```python
from build123d import *

# Parameters (mm, degrees)
SKETCH_1_R      = 33
SKETCH_1_R_2    = 4
SKETCH_1_R_3    = 7
EXTRUDE_1_DEPTH = 10
SKETCH_1_3_R    = 33
EXTRUDE_2_DEPTH = 20


with BuildPart() as part:
    # Sketch 1 → Extrude 1 (new body)
    with BuildSketch(Plane.XY):
        with BuildLine():
            ThreePointArc((64, -136), (75.313708499, -140.686291501), (80, -152))
            Line((80, -152), (27.5, -152))
            Line((27.5, -152), (14.463080892, -104.593021426))
            ThreePointArc((14.463080892, -104.593021426), (0, -93.570368671), (-14.463080892, -104.593021426))
            Line((-14.463080892, -104.593021426), (-27.5, -152))
            Line((-27.5, -152), (-80, -152))
            ThreePointArc((-80, -152), (-75.313708499, -140.686291501), (-64, -136))
            Line((-64, -136), (-60.459937025, -136))
            ThreePointArc((-60.459937025, -136), (-51.367638325, -132.930218118), (-45.996856133, -124.977347245))
            Line((-45.996856133, -124.977347245), (-29.300488581, -64.26328342))
            ThreePointArc((-29.300488581, -64.26328342), (-29.160343249, -48.882298429), (-36.661224304, -35.453555993))
            ThreePointArc((-36.661224304, -35.453555993), (-48.195333852, -16.679622146), (-50.733420691, 5.207689026))
            ThreePointArc((-50.733420691, 5.207689026), (-51.500326923, 13.089309145), (-55.266020254, 20.05548705))
            ThreePointArc((-55.266020254, 20.05548705), (-51.548317959, 55.688646816), (-16.027753707, 51.016077878))
            ThreePointArc((-16.027753707, 51.016077878), (0, 42.978983508), (16.027753707, 51.016077878))
            ThreePointArc((16.027753707, 51.016077878), (51.548317959, 55.688646816), (55.266020254, 20.05548705))
            ThreePointArc((55.266020254, 20.05548705), (51.500326923, 13.089309145), (50.733420691, 5.207689026))
            ThreePointArc((50.733420691, 5.207689026), (48.195333852, -16.679622146), (36.661224304, -35.453555993))
            ThreePointArc((36.661224304, -35.453555993), (29.160343249, -48.882298429), (29.300488581, -64.26328342))
            Line((29.300488581, -64.26328342), (45.996856133, -124.977347245))
            ThreePointArc((45.996856133, -124.977347245), (51.367638325, -132.930218118), (60.459937025, -136))
            Line((60.459937025, -136), (64, -136))
        make_face()
        Circle(SKETCH_1_R, mode=Mode.SUBTRACT)
        with Locations((40.203550562, 20.60763262)):
            Circle(SKETCH_1_R_2, mode=Mode.SUBTRACT)
        with Locations((36.062445841, 36.062445841)):
            Circle(SKETCH_1_R_3, mode=Mode.SUBTRACT)
        with Locations((-36.062445841, 36.062445841)):
            Circle(SKETCH_1_R_3, mode=Mode.SUBTRACT)
        with Locations((-47.376154339, 47.376154339)):
            Circle(SKETCH_1_R_2, mode=Mode.SUBTRACT)
        with Locations((-20.60763262, 40.203550562)):
            Circle(SKETCH_1_R_2, mode=Mode.SUBTRACT)
        with Locations((-40.203550562, 20.60763262)):
            Circle(SKETCH_1_R_2, mode=Mode.SUBTRACT)
        with Locations((47.376154339, 47.376154339)):
            Circle(SKETCH_1_R_2, mode=Mode.SUBTRACT)
        with Locations((20.60763262, 40.203550562)):
            Circle(SKETCH_1_R_2, mode=Mode.SUBTRACT)
    extrude(amount=EXTRUDE_1_DEPTH)

    # Sketch 1_3 → Extrude 2 (add)
    with BuildSketch(Plane.XY):
        Circle(SKETCH_1_3_R)
        with BuildLine():
            ThreePointArc((4, -16.522711642), (7.376023565, -15.316470754), (10.42401693, -13.429068138))
            Line((10.42401693, -13.429068138), (16.007550501, -17.881787577))
            Line((16.007550501, -17.881787577), (20.995468916, -11.627135717))
            Line((20.995468916, -11.627135717), (15.411935345, -7.174416278))
            ThreePointArc((15.411935345, -7.174416278), (16.573774507, -3.782855877), (16.9985365, -0.223062423))
            Line((16.9985365, -0.223062423), (23.961088981, 1.366094746))
            Line((23.961088981, 1.366094746), (22.180921509, 9.165518044))
            Line((22.180921509, 9.165518044), (15.218369029, 7.576360875))
            ThreePointArc((15.218369029, 7.576360875), (13.291135202, 10.599326632), (10.772811379, 13.150913846))
            Line((10.772811379, 13.150913846), (13.87143874, 19.585279862))
            Line((13.87143874, 19.585279862), (6.663687797, 23.056349775))
            Line((6.663687797, 23.056349775), (3.565060436, 16.621983759))
            ThreePointArc((3.565060436, 16.621983759), (0, 17), (-3.565060436, 16.621983759))
            Line((-3.565060436, 16.621983759), (-6.663687797, 23.056349775))
            Line((-6.663687797, 23.056349775), (-13.87143874, 19.585279862))
            Line((-13.87143874, 19.585279862), (-10.772811379, 13.150913846))
            ThreePointArc((-10.772811379, 13.150913846), (-13.291135202, 10.599326632), (-15.218369029, 7.576360875))
            Line((-15.218369029, 7.576360875), (-22.180921509, 9.165518044))
            Line((-22.180921509, 9.165518044), (-23.961088981, 1.366094746))
            Line((-23.961088981, 1.366094746), (-16.9985365, -0.223062423))
            ThreePointArc((-16.9985365, -0.223062423), (-16.573774507, -3.782855877), (-15.411935345, -7.174416278))
            Line((-15.411935345, -7.174416278), (-20.995468916, -11.627135717))
            Line((-20.995468916, -11.627135717), (-16.007550501, -17.881787577))
            Line((-16.007550501, -17.881787577), (-10.42401693, -13.429068138))
            ThreePointArc((-10.42401693, -13.429068138), (-7.376023565, -15.316470754), (-4, -16.522711642))
            Line((-4, -16.522711642), (-4, -23.664319132))
            Line((-4, -23.664319132), (4, -23.664319132))
            Line((4, -23.664319132), (4, -16.522711642))
        make_face(mode=Mode.SUBTRACT)
    extrude(amount=EXTRUDE_2_DEPTH)


solid = part.part
```
Geometry check sheet. Reference: the model listing, model coordinates, mm. A direction names the side the tool comes from. Give positions to 0.01 mm unless a question says otherwise; leave off trailing zeros. Loops run counter-clockwise (first coordinate to the right, second up) from the corner with the lowest first, then second, coordinate; pieces in that order, holes last. Notation, with made-up numbers: M -15.75,-9 L 10.25,-9 A21 cw 10.25,27 Z; hole C 76.25,46.25 d5. An arc over 180 degrees is marked long. Write item = value, one per line. Start each with the question number.
1. Section check B-B, the plane x = -40. Enter the section's corners in (y, z), plus the area to 3 significant figures.
2. Section check A-A, the plane x = 0. Enter the section's corners in (y, z).
3. Section check D-D, the plane y = -62. Enter the section's corners in (x, z).
4. Section check C-C, the plane z = 5.5. Give the number of separate pieces and of enclosed holes in the cut face, plus the area to 3 significant figures.
5. Draft check along Y on faces 4 (the face through (-75.437, -140.811, 4.93)), 5 (the face through (22, 0, 20)), 6 (the face through (51.07, 45.84, 4.93)). Enter one of: +Y half, -Y half, draft (parallel to the pull), parting line (faces both ways), or undercut.
6. Go/stop test with flat-tipped pins: P1, Ø5, axis at y = -67, z = 9, coming from the -X side; P2, Ø13, axis at x = 20.61, y = 40.2, coming from the +Z side; P3, Ø5.5, axis at y = -18.5, z = 11.5, coming from the +X side. Record where each tip stops, or that it passes through.
7. Thickness scan on probe 1 along Y at (x, z) = (-0.5, 4.75); probe 2 along Y at (x, z) = (11.5, 13); probe 3 along X at (y, z) = (-0.5, 17.75). Record the ranges inside material, lowest first.
8. Tool access check on faces 1 (the face through (5.136, 19.884, 9.86)), 2 (the face through (0.273, -93.573, 4.93)), 3 (the face through (-51.477, -133.013, 4.93)). Record the directions out of +Z, -Z, +X, -X, +Y, -Y that give a thin tool (end or side, any length) a straight path to the whole face; none if there is none.
Values follow:
q1.outline = M -152,0 L -103.17,0 L -103.17,10 L -152,10 Z; M -31.64,0 L 16.61,0 L 16.61,10 L -31.64,10 Z; M 24.6,0 L 30.27,0 L 30.27,10 L 24.6,10 Z; M 41.85,0 L 60.75,0 L 60.75,10 L 41.85,10 Z
q1.area = 1,220 mm^2
q2.outline = M -93.57,0 L -23.66,0 L -23.66,20 L -33,20 L -33,10 L -93.57,10 Z; M 17,0 L 42.98,0 L 42.98,10 L 33,10 L 33,20 L 17,20 Z
q3.outline = M -28.77,0 L 28.77,0 L 28.77,10 L -28.77,10 Z
q4.separate_pieces = 1
q4.enclosed_holes = 9
q4.area = 15,200 mm^2
q5.face_4 = +Y half
q5.face_5 = draft
q5.face_6 = undercut
q6.P1 = -30.74
q6.P2 = 10
q6.P3 = 48.36
q7.probe_1 = -93.58 to -23.66, 16.99 to 42.99
q7.probe_2 = -30.93 to -14.29, 12.52 to 14.66, 20.73 to 30.93
q7.probe_3 = -33 to -16.99, 16.99 to 33
q8.face_1 = +Z, -Z
q8.face_2 = +Z, -Z, -Y
q8.face_3 = +Z, -Z, -X
